Geometry check sheet. Reference: the model listing, model coordinates, mm. A direction names the side the tool comes from. Round coordinates to 2 decimals unless told otherwise and drop trailing zeros. Order: outer loops, then holes, each group sorted by start corner. A loop starts at its lowest first (then second) coordinate and runs counter-clockwise, first axis right, second up.
(1) Set-up check for faces 3 (the face through (4.5, 0, 0)), 4 (the face through (0, 0, -0.1)): record each of +Z, -Z, +X, -X, +Y, -Y from which the full face is reachable in a straight line by a thin tool's end or side.
(2) Release check for a two-part mould opening along Z. For faces 1 (the face through (-4.5, 0, 0)), 2 (the face through (-4, -0.2, -0.5)) record: +Z half, -Z half, draft (parallel to the pull), parting line (faces both ways), or undercut.
(3) Sectioned sample at B-B (y = -12.5). Record the boundary of the cut face in (x, z).
(4) Material ranges on line 1 along X through (y, z) = (-5.75, 0.2), recorded low to high.
(5) Sectioned sample at A-A (z = -0.45). Record the boundary of the cut face in (x, y).
(6) Sectioned sample at C-C (x = 3.5). Record the boundary of the cut face in (y, z).
from build123d import *

# Parameters (mm, degrees)
SKETCH1_W           = 9
SKETCH1_H           = 2
BOSS_EXTRUDE1_DEPTH = 15
CUT_EXTRUDE1_START  = -31
SKETCH2_W           = 8
SKETCH2_H           = 0.8
CUT_EXTRUDE1_DEPTH  = 32


with BuildPart() as part:
    # Sketch1 → Boss-Extrude1 (new body, symmetric)
    with BuildSketch(Plane(origin=(0, 0, 0), x_dir=(1, 0, 0), z_dir=(0, 1, 0))):
        Rectangle(SKETCH1_W, SKETCH1_H)
    extrude(amount=BOSS_EXTRUDE1_DEPTH, both=True)

    # Sketch2 → Cut-Extrude1 (cut)
    with BuildSketch(Plane(origin=(0, 15, 0), x_dir=(1, 0, 0), z_dir=(0, 1, 0)).offset(CUT_EXTRUDE1_START)):
        with Locations((0, 0.5)):
            Rectangle(SKETCH2_W, SKETCH2_H)
    cut_extrude1 = extrude(amount=CUT_EXTRUDE1_DEPTH, mode=Mode.SUBTRACT)

    # Mirror1: Cut-Extrude1 across plane
    add(cut_extrude1.mirror(Plane.XY), mode=Mode.SUBTRACT)


solid = part.part
Answer below:
1. face 3: +Z, -Z, +X, +Y, -Y
1. face 4: +Y, -Y
2. face 1: draft
2. face 2: undercut
3. outline: (-4.5, -1) - (4.5, -1) - (4.5, 1) - (-4.5, 1) - close; hole (-4, -0.9) - (4, -0.9) - (4, -0.1) - (-4, -0.1) - close; hole (-4, 0.1) - (4, 0.1) - (4, 0.9) - (-4, 0.9) - close
4. line 1: x = -4.5 to -4, 4 to 4.5
5. outline: (-4.5, -15) - (-4, -15) - (-4, 15) - (-4.5, 15) - close; (4, -15) - (4.5, -15) - (4.5, 15) - (4, 15) - close
6. outline: (-15, -1) - (15, -1) - (15, -0.9) - (-15, -0.9) - close; (-15, -0.1) - (15, -0.1) - (15, 0.1) - (-15, 0.1) - close; (-15, 0.9) - (15, 0.9) - (15, 1) - (-15, 1) - close
